The drawing under review shows one solid part. Ordinate dimensions are in mm from its lowest x, y, z. A direction names the side the tool comes from. Coordinates: 2 decimals unless noted, no trailing zeros. Order: outer loops, then holes, each group sorted by start corner. A loop starts at its lowest first (then second) coordinate and runs counter-clockwise, first axis right, second up.
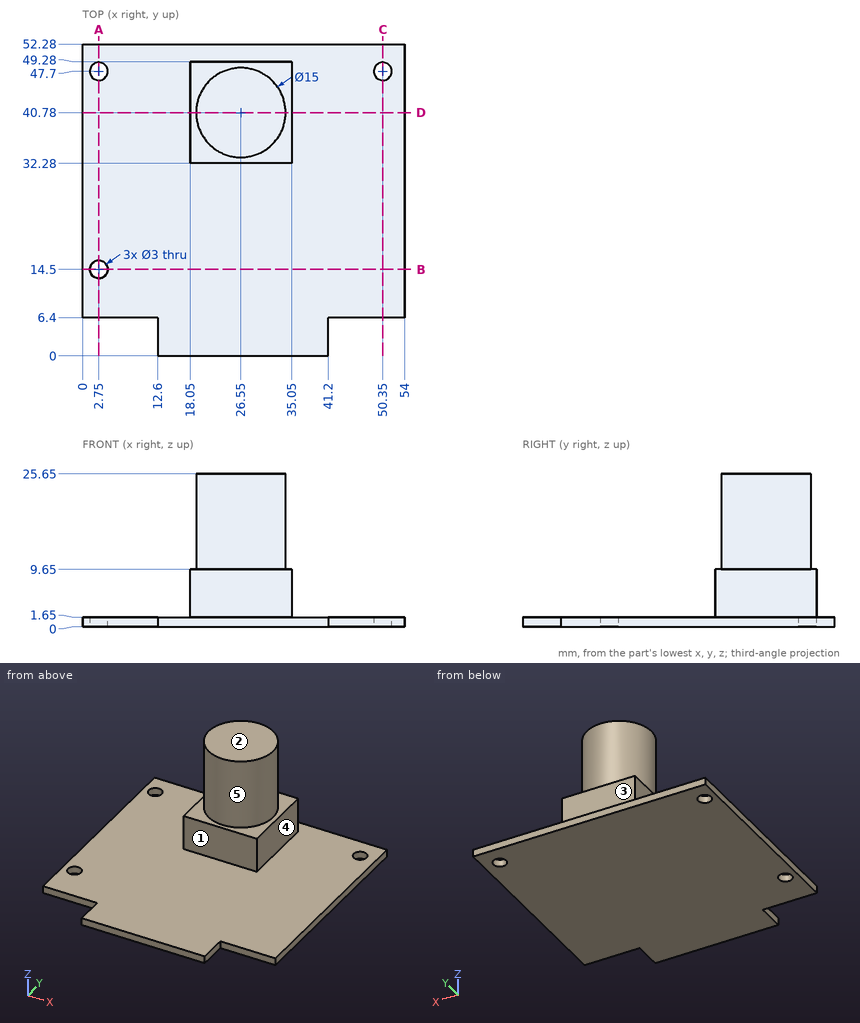
(1) Machinability: for the marked faces 1, 2, 3, 4 and 5, which of the approach directions +Z, -Z, +X, -X, +Y, -Y give a long, thin tool a straight path to every point of the face, cutting with its end or side? Answer none if there is none.
A:
face 1: +Z, +X, -X, -Y
face 2: +Z, +X, -X, +Y, -Y
face 3: +Z, +X, -X, +Y
face 4: +Z, +X, +Y, -Y
face 5: +Z
(2) For pin 1 Ø4 at (y, z) = (37.5, 6.5) entering from -X; pin 2 Ø12 at (x, z) = (27.5, 10.5) entering from +Y; pin 3 Ø0.8 at (y, z) = (2, 1) entering from -X, all flat-tipped, find the tip position at first contact; note any pin that passes through.
A:
pin 1: stops at x = 18.05
pin 2: stops at y = 49.28
pin 3: stops at x = 12.6
(3) We need section C-C, the plane x = 50.35. Write out the cut boundary in (y, z), and give its area (3 significant figures).
A:
outline: (6.4, 0) - (46.2, 0) - (46.2, 1.65) - (6.4, 1.65) - close; (49.2, 0) - (52.28, 0) - (52.28, 1.65) - (49.2, 1.65) - close
area: 70.8 mm2
(4) Wall thickness on probe 1 along Y at (x, z) = (50.35, 0.9); probe 2 along X at (y, z) = (14.5, 0.5); probe 3 along Z at (x, y) = (13.5, 8): over which ranges is each line inside the solid? List them lowest first.
A:
probe 1: y = 6.4 to 46.2, 49.2 to 52.28
probe 2: x = 0 to 1.25, 4.25 to 54
probe 3: z = 0 to 1.65
(5) We need section D-D, the plane y = 40.78. Write out the cut boundary in (x, z).
A:
outline: (0, 0) - (54, 0) - (54, 1.65) - (35.05, 1.65) - (35.05, 9.65) - (34.05, 9.65) - (34.05, 25.65) - (19.05, 25.65) - (19.05, 9.65) - (18.05, 9.65) - (18.05, 1.65) - (0, 1.65) - close
(6) We need section A-A, the plane x = 2.75. Write out the cut boundary in (y, z).
A:
outline: (6.4, 0) - (13, 0) - (13, 1.65) - (6.4, 1.65) - close; (16, 0) - (46.2, 0) - (46.2, 1.65) - (16, 1.65) - close; (49.2, 0) - (52.28, 0) - (52.28, 1.65) - (49.2, 1.65) - close
(7) We need section B-B, the plane y = 14.5. Write out the cut boundary in (x, z), and give its area (4 significant figures).
A:
outline: (0, 0) - (1.25, 0) - (1.25, 1.65) - (0, 1.65) - close; (4.25, 0) - (54, 0) - (54, 1.65) - (4.25, 1.65) - close
area: 84.15 mm2
